Model file for the job. Use its own axes, mm. Face numbers are marked on the shaded views. Give positions to 0.01 mm unless a question says otherwise; leave off trailing zeros. Order: outer loops, then holes, each group sorted by start corner. A loop starts at its lowest first (then second) coordinate and runs counter-clockwise, first axis right, second up. Notation, with made-up numbers: M 59.5,89 L 108.5,89 A10 cw 108.5,97 Z; hole C 86.25,55 d4. An arc over 180 degrees is marked long. Return JSON: item names as keys, results as strings. Group by question number.
1. Two-plate mould, pull along X, no slides. Class the marked faces 1, 2 and 3: released by +X, released by -X, zero draft, split by the parting line, or undercut.
2. Slice it at D-D on x = -1. List the corners of the cut face in (y, z) (3 decimals).
3. Slice it at A-A on z = 118. List the corners of the cut face in (x, y) (3 decimals).
4. Slice it at C-C on z = 40.5. List the corners of the cut face in (x, y).
5. Pin check, flat tips, straight feed: pin 1 (16 mm diameter, centred on x = -10.5, z = 32.5, fed in from +Y); pin 2 (3 mm diameter, centred on x = -22.5, y = 4.5, fed in from +Z) (3 decimals); pin 3 (9.5 mm diameter, centred on y = 8, z = 31, fed in from +X). Stop position of each tip, or through.
6. Slice it at B-B on y = 22.5. List the corners of the cut face in (x, z) (3 decimals), then the cut area to 3 significant figures.
7. Wall check: probe 1 along X at (y, z) = (-34.5, 197.5) (3 decimals); probe 2 along Y at (x, z) = (-20.5, 45.5); probe 3 along Z at (x, y) = (28.5, -26) (3 decimals). Give the ranges that are in metal, low to high. Write a range as [from, to].
from build123d import *

# Parameters (mm, degrees)
F1_DEPTH  = 38.1
F2_W      = 71.12
F2_H      = 27.3908400369
F3_DEPTH  = 50.8
F4_W      = 25.4
F4_H      = 19.05
F5_DEPTH  = 190.5
F6_W      = 12.7
F6_H      = 152.4
F7_DEPTH  = 6.35
F9_DEPTH  = 6.35
F10_R     = 8.0648205789
F11_DEPTH = 76.2
F13_DEPTH = 76.2
F15_DEPTH = 6.35
F17_DEPTH = 6.35
F18_W     = 6.35
F18_H     = 146.05
F19_DEPTH = 25.4


with BuildPart() as f1:
    # F0 (on Front) → F1 (new body, symmetric)
    with BuildSketch(Plane.XZ):
        Polygon((30.48, -22.225), (49.53, -22.225), (49.53, 22.225), (-49.53, 22.225), (-49.53, -22.225), (-30.48, -22.225), (-30.48, 3.175), (30.48, 3.175), align=None)
    extrude(amount=F1_DEPTH, both=True)

    # F2 (on Front) → F3 (cut, symmetric)
    with BuildSketch(Plane.XZ):
        with Locations((0, -23.2204200185)):
            Rectangle(F2_W, F2_H)
    extrude(amount=F3_DEPTH, both=True, mode=Mode.SUBTRACT)

    # F4 (on face) → F5 (join)
    with BuildSketch(Plane.XY.offset(22.225)):
        with Locations((-36.83, -28.575)):
            Rectangle(F4_W, F4_H)
    extrude(amount=F5_DEPTH)

    # F6 (on face) → F7 (cut)
    with BuildSketch(Plane(origin=(0, -19.05, 0), x_dir=(-1, 0, 0), z_dir=(0, 1, 0))):
        with Locations((36.83, 136.525)):
            Rectangle(F6_W, F6_H)
    extrude(amount=-F7_DEPTH, mode=Mode.SUBTRACT)

    # F8 (on face) → F9 (cut)
    with BuildSketch(Plane(origin=(0, -19.05, 0), x_dir=(-1, 0, 0), z_dir=(0, 1, 0))):
        Polygon((33.655, 200.025), (33.655, 225.425), (20.955, 225.425), (20.955, 200.025), (24.13, 200.025), (24.13, 212.725), (30.48, 212.725), (30.48, 200.025), align=None)
    extrude(amount=-F9_DEPTH, mode=Mode.SUBTRACT)

    # F10 (on face) → F11 (join)
    with BuildSketch(Plane.XZ.offset(38.1)):
        with Locations((-35.56, -9.525)):
            Circle(F10_R)
    extrude(amount=-F11_DEPTH)

    # F12 (on face) → F13 (join)
    with BuildSketch(Plane.XZ.offset(38.1)):
        Polygon((35.56, -17.4720194191), (35.56, -9.525), (30.48, -9.525), align=None)
    extrude(amount=-F13_DEPTH)

    # F14 (on face) → F15 (join)
    with BuildSketch(Plane.XZ.offset(38.1)):
        Polygon((-24.13, 53.975), (-24.13, 22.225), (13.97, 22.225), align=None)
    extrude(amount=-F15_DEPTH)

    # F16 (on face) → F17 (join)
    with BuildSketch(Plane(origin=(-49.53, 0, 0), x_dir=(0, -1, 0), z_dir=(-1, 0, 0))):
        Polygon((-19.05, 22.225), (19.05, 22.225), (19.05, 53.975), align=None)
    extrude(amount=-F17_DEPTH)

    # F18 (on face) → F19 (cut)
    with BuildSketch(Plane.XZ.offset(38.1)):
        with Locations((-36.83, 133.35)):
            Rectangle(F18_W, F18_H)
    extrude(amount=-F19_DEPTH, mode=Mode.SUBTRACT)


solid = f1.part
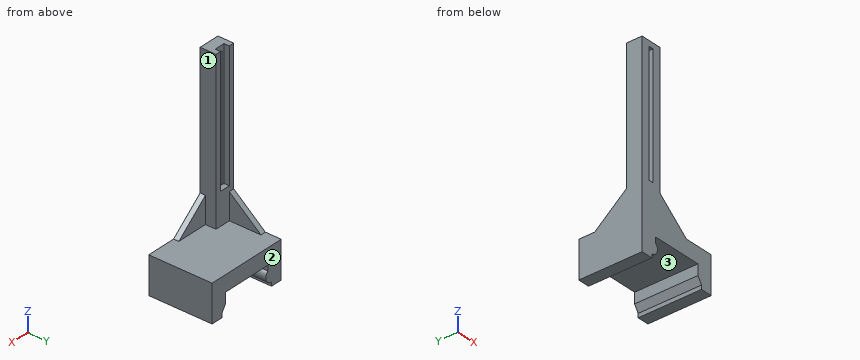
Result:
{
 "1": {"face 1": "released by +X", "face 2": "zero draft", "face 3": "undercut"},
 "2": {"outline": "M -38.1,3.175 L 38.1,3.175 L 38.1,22.225 L -31.75,22.225 L -31.75,34.7 L -38.1,34.7 Z"},
 "3": {"outline": "M -49.53,-38.1 L -40.005,-38.1 L -40.005,-25.4 L -43.18,-25.4 L -43.18,-19.05 L -49.53,-19.05 Z; M -33.655,-38.1 L -24.13,-38.1 L -24.13,-19.05 L -30.48,-19.05 L -30.48,-25.4 L -33.655,-25.4 Z"},
 "4": {"outline": "M -49.53,-38.1 L -7.96,-38.1 L -7.96,-31.75 L -24.13,-31.75 L -24.13,-19.05 L -43.18,-19.05 L -43.18,-2.88 L -49.53,-2.88 Z"},
 "5": {"pin 1": "stops at y = -31.75", "pin 2": "stops at z = 22.225", "pin 3": "stops at x = -43.18"},
 "6": {"outline": "M -49.53,-22.225 L -35.56,-22.225 L -35.56,-17.59 A8.065 ccw -30.48,-3.261 L -30.48,3.175 L 30.48,3.175 L 30.48,-9.525 L 35.56,-17.472 L 35.56,-22.225 L 49.53,-22.225 L 49.53,22.225 L -49.53,22.225 Z", "area": "2,810 mm2"},
 "7": {"probe 1": "x = [-49.53, -40.005], [-33.655, -24.13]", "probe 2": "y = [-38.1, -31.75]", "probe 3": "z = [3.175, 22.225]"}
}
